Can you work these out from the model? Positions are in its coordinate system, mm. Give positions to 0.01 mm unless a question says otherwise; leave off trailing zeros. Order: outer loops, then holes, each group sorted by start corner. A loop starts at its lowest first (then second) coordinate and runs counter-clockwise, first axis right, second up. Notation, with made-up numbers: M -34.75,82.5 L 7.25,82.5 A28 ccw 7.25,109.5 Z; hole C -37,45.25 d3. An arc over 180 degrees is marked long. Answer as a JSON object with one key per item and string values.
```python
from build123d import *

# Parameters (mm, degrees)
F0_W            = 50
F0_H            = 8
F1_DEPTH        = 4
F3_DEPTH        = 5
F4_DEPTH        = 5
F5_D            = 3.3
F5_CBORE_D      = 6.5
F5_CBORE_DEPTH  = 0
F6_DEPTH        = 1.1
F7_DEPTH        = 4.4
F8_DEPTH        = 3.5
F9_DEPTH        = 8.7
F11_D           = 3.3
F11_CBORE_D     = 6.5
F11_CBORE_DEPTH = 0


with BuildPart() as f1:
    # F0 (on Top) → F1 (new body)
    with BuildSketch(Plane.XY):
        Rectangle(F0_W, F0_H)
    extrude(amount=F1_DEPTH)

    # F3 (add): a face of the model
    f3_faces = [f1.faces().sort_by_distance(p)[0] for p in [
        (0, -4, 2),
    ]]
    extrude(f3_faces, amount=F3_DEPTH)

    # F4 (add): a face of the model
    f4_faces = [f1.faces().sort_by_distance(p)[0] for p in [
        (0, 4, 2),
    ]]
    extrude(f4_faces, amount=F4_DEPTH)

    # F5 (through all)
    with Locations(Plane.XY.offset(4)):
        with Locations((0, -4)):
            CounterBoreHole(F5_D / 2, F5_CBORE_D / 2, F5_CBORE_DEPTH)

    # F6 (cut): a face of the model
    f6_faces = [f1.faces().sort_by_distance(p)[0] for p in [
        (0, -9, 2),
    ]]
    extrude(f6_faces, amount=-F6_DEPTH, mode=Mode.SUBTRACT)

    # F7 (add): a face of the model
    f7_faces = [f1.faces().sort_by_distance(p)[0] for p in [
        (0, 9, 2),
    ]]
    extrude(f7_faces, amount=F7_DEPTH)

    # F8 (cut): a face of the model
    f8_faces = [f1.faces().sort_by_distance(p)[0] for p in [
        (0, 2.8046479423, 0),
    ]]
    extrude(f8_faces, amount=-F8_DEPTH, mode=Mode.SUBTRACT)

    # F9 (add): a face of the model
    f9_faces = [f1.faces().sort_by_distance(p)[0] for p in [
        (0, 13.4, 3.75),
    ]]
    extrude(f9_faces, amount=F9_DEPTH)

    # F11 (through all)
    with Locations(Plane.XY.offset(4)):
        with Locations((-18, 17.4584981568), (18, 17.4584981568)):
            CounterBoreHole(F11_D / 2, F11_CBORE_D / 2, F11_CBORE_DEPTH)


solid = f1.part
```
1) I need wall thicknesses on L1, parallel to Y at x = 0, z = 3.85; L2, parallel to X at y = 18.5, z = 3.9; L3, parallel to Y at x = -18, z = 3.8. Which ranges of each line are inside material? Lowest first, please.
Results found:
{"L1": "y = -7.9 to -5.65, -2.35 to 22.1", "L2": "x = -25 to -19.28, -16.72 to 16.72, 19.28 to 25", "L3": "y = -7.9 to 15.81, 19.11 to 22.1"}
2) I want a section at C-C on z = 3.6. Write out the boundary of the cut face in (x, y).
Results found:
{"outline": "M -25,-7.9 L 25,-7.9 L 25,22.1 L -25,22.1 Z; hole C -18,17.46 d3.3; hole C 0,-4 d3.3; hole C 18,17.46 d3.3"}
3) I want a section at B-B on x = -18. Write out the boundary of the cut face in (y, z), and give its area (4 significant figures).
Results found:
{"outline": "M -7.9,3.5 L 15.81,3.5 L 15.81,4 L -7.9,4 Z; M 19.11,3.5 L 22.1,3.5 L 22.1,4 L 19.11,4 Z", "area": "13.35 mm²"}
4) Thinking about a two-plate mould opening in X: for faces 1 (the face through (0, 7, 4)), 2 (the face through (19.22, 18.57, 3.75)), 3 (the face through (0.4, -5.6, 3.7)), which applies, pulls with the +X half, pulls with the -X half, needs draft (parallel to the pull), parting line crosses it, or undercut?
Results found:
{"face 1": "needs draft", "face 2": "undercut", "face 3": "undercut"}
5) I want a section at A-A on y = -4. Write out the boundary of the cut face in (x, z), and give its area (4 significant figures).
Results found:
{"outline": "M -25,3.5 L -1.65,3.5 L -1.65,4 L -25,4 Z; M 1.65,3.5 L 25,3.5 L 25,4 L 1.65,4 Z", "area": "23.35 mm²"}
